from build123d import *

# Parameters (mm, degrees)
F0_R     = 2.6
F0_W     = 5.2
F0_H     = 2.5
F1_DEPTH = 6
F2_R     = 1.5
F3_R     = 1


with BuildPart() as f1:
    # F0 (on Top) → F1 (new body)
    with BuildSketch(Plane.XY):
        with BuildLine():
            ThreePointArc((3.196213, 1.25), (4.526647, 2.971475), (5, 5.095026))
            ThreePointArc((5, 5.095026), (-2.123551, 9.621673), (-3.196213, 1.25))
            ThreePointArc((-3.196213, 1.25), (0, 0.095026), (3.196213, 1.25))
        make_face()
        with Locations((0, 5.095026)):
            Circle(F0_R, mode=Mode.SUBTRACT)
        with BuildLine():
            ThreePointArc((3.196213, 1.25), (0, 0.095026), (-3.196213, 1.25))
            Line((-3.196213, 1.25), (-3.196213, 0))
            Line((-3.196213, 0), (0, 0))
            Line((0, 0), (3.196213, 0))
            Line((3.196213, 0), (3.196213, 1.25))
        make_face()
        with BuildLine():
            Line((0, 0), (-3.196213, 0))
            Line((-3.196213, 0), (-3.196213, -1.25))
            ThreePointArc((-3.196213, -1.25), (0, -0.095026), (3.196213, -1.25))
            Line((3.196213, -1.25), (3.196213, 0))
            Line((3.196213, 0), (0, 0))
        make_face()
        with BuildLine():
            ThreePointArc((3.196213, -1.25), (0, -0.095026), (-3.196213, -1.25))
            ThreePointArc((-3.196213, -1.25), (-2.123551, -9.621673), (5, -5.095026))
            ThreePointArc((5, -5.095026), (4.526647, -2.971475), (3.196213, -1.25))
        make_face()
        with Locations((0, -4.595026)):
            Rectangle(F0_W, F0_H, mode=Mode.SUBTRACT)
    extrude(amount=F1_DEPTH)

    # F2
    f2_edges = [f1.edges().sort_by_distance(p)[0] for p in [
        (0, -5.845026, 6),
        (0, -5.845026, 0),
    ]]
    fillet(f2_edges, radius=F2_R)

    # F3
    f3_edges = [f1.edges().sort_by_distance(p)[0] for p in [
        (-3.196213, 0, 6),
        (0, 10.095026, 6),
        (3.196213, 0, 6),
        (0, -10.095026, 6),
        (0, 10.095026, 0),
        (3.196213, 0, 0),
        (-3.196213, 0, 0),
        (0, -10.095026, 0),
    ]]
    fillet(f3_edges, radius=F3_R)


solid = f1.part
Check sheet for the modelled part. Datum: model origin and axes. Units: mm. A direction names the side the tool comes from. Give positions to 0.01 mm unless a question says otherwise; leave off trailing zeros. Loops run counter-clockwise (first coordinate to the right, second up) from the corner with the lowest first, then second, coordinate; pieces in that order, holes last. Notation, with made-up numbers: M 28,48.5 L 47,48.5 A5 cw 47,56.5 Z; hole C 59,-7 d5. An arc over 180 degrees is marked long. Answer as a JSON object with one key per item and string values. Group by question number.
Q1. Material ranges on line 1 along Y through (x, z) = (0, 1.55); line 2 along Y through (x, z) = (0, 4.8); line 3 along X through (y, z) = (3.75, 3.5), recorded low to high. Write a range as [from, to].
Q2. Release check for a two-part mould opening along X. For faces 4 (the cylindrical face through (-2.9, -0.02, 0.29)), 5 (the cylindrical face through (0.036, -6.273, 0.451)), 6 (the flat face through (3.196, 0, 3)) record: released by +X, released by -X, zero draft, split by the parting line, or undercut.
Q3. Go/stop test with flat-tipped pins: P1, Ø2, axis at y = -6, z = 4, coming from the -X side; P2, Ø1, axis at y = 6.5, z = 1.5, coming from the -X side; P3, Ø1.2, axis at y = 0, z = 2, coming from the +X side; P4, Ø2, axis at y = -0.5, z = 4, coming from the -X side (3 decimals). Record where each tip stops, or that it passes through.
Q4. Cross-section at A-A on z = 5.75. Record the cut outline in (x, y).
Q5. Access from +Z, -Z, +X, -X, +Y, -Y to the whole of each face (thin tool, end or side, straight path). Record for faces 1 (the flat face through (-3.196, 0, 3)), 2 (the cylindrical face through (-2.91, -0.02, 5.7)), 3 (the cylindrical face through (2.91, 0.02, 5.7)).
Q6. Cross-section at B-B on x = 0. Give the number of separate pieces and of enclosed holes in the cut face, then the cut area to 3 significant figures.
Evaluation:
{
 "1": {"line 1": "y = [-10.1, -5.85], [-3.35, 2.5], [7.7, 10.1]", "line 2": "y = [-10.1, -5.88], [-3.35, 2.5], [7.7, 10.1]", "line 3": "x = [-4.82, -2.23], [2.23, 4.82]"},
 "2": {"face 4": "released by -X", "face 5": "undercut", "face 6": "released by +X"},
 "3": {"P1": "stops at x = -5", "P2": "stops at x = -4.92", "P3": "stops at x = 3.2", "P4": "stops at x = -3.475"},
 "4": {"outline": "M -2.86,-1.41 A4.66 ccw long 2.86,-1.41 L 2.86,1.41 A4.66 ccw long -2.86,1.41 Z; hole M -2.6,-6.52 L 2.6,-6.52 L 2.6,-3.35 L -2.6,-3.35 Z; hole C 0,5.1 d5.2"},
 "5": {"face 1": "+Z, -Z, -X", "face 2": "+Z, -X", "face 3": "+Z, +X"},
 "6": {"separate pieces": "3", "enclosed holes": "0", "area": "73.1 mm2"}
}
